from build123d import *

# Parameters (mm, degrees)
EXTRUDE_1_DEPTH      = 40
EXTRUDE_1_DEPTH_BACK = 5
SKETCH_2_W           = 36
SKETCH_2_H           = 37
CUT_EXTRUDE_1_DEPTH  = 50
SKETCH_5_W           = 36
SKETCH_5_H           = 5
CUT_EXTRUDE_4_DEPTH  = 43
SKETCH_9_R           = 1.025
CUT_EXTRUDE_5_DEPTH  = 45.5
SKETCH_10_W          = 3
SKETCH_10_H          = 8
EXTRUDE_4_DEPTH      = 10
SKETCH_11_W          = 3
SKETCH_11_H          = 18.5
EXTRUDE_5_DEPTH      = 10
SKETCH_12_R          = 1.05
CUT_EXTRUDE_6_DEPTH  = 10
SKETCH_13_R          = 1.05
CUT_EXTRUDE_7_DEPTH  = 63.5
FILLET_4_R           = 2
FILLET_5_R           = 2
FILLET_6_R           = 2
FILLET_7_R           = 2


with BuildPart() as part:
    # 草圖1 → 填料-伸長1 (new, two sides: drawn at the far end of the back side and taken through both)
    with BuildSketch(Plane.XY.offset(-EXTRUDE_1_DEPTH_BACK)):
        Polygon((-14.545454545, -28.090909091), (-15.545454545, -28.090909091), (-15.545454545, 16.909090909), (-14.545454545, 16.909090909), (25.454545455, 16.909090909), (26.454545455, 16.909090909), (26.454545455, -28.090909091), (25.454545455, -28.090909091), align=None)
    extrude(amount=EXTRUDE_1_DEPTH + EXTRUDE_1_DEPTH_BACK)

    # 草圖2 → 除料-伸長1 (cut)
    with BuildSketch(Plane(origin=(0, 16.909090909, 0), x_dir=(1, 0, 0), z_dir=(0, 1, 0))):
        with Locations((5.454545455, -21.5)):
            Rectangle(SKETCH_2_W, SKETCH_2_H)
    extrude(amount=-CUT_EXTRUDE_1_DEPTH, mode=Mode.SUBTRACT)

    # 草圖5 → 除料-伸長4 (cut)
    with BuildSketch(Plane(origin=(0, 16.909090909, 0), x_dir=(1, 0, 0), z_dir=(0, 1, 0))):
        with Locations((5.454545455, -0.5)):
            Rectangle(SKETCH_5_W, SKETCH_5_H)
    extrude(amount=-CUT_EXTRUDE_4_DEPTH, mode=Mode.SUBTRACT)

    # 草圖9 → 除料-伸長5 (cut)
    with BuildSketch(Plane.ZY.offset(15.545454545)):
        with Locations(Location((37, -25.090909091, 0), (0, 0, 180))):
            Circle(SKETCH_9_R)
        with Locations(Location((37, 13.909090909, 0), (0, 0, 180))):
            Circle(SKETCH_9_R)
    extrude(amount=-CUT_EXTRUDE_5_DEPTH, mode=Mode.SUBTRACT)

    # 草圖10 → 填料-伸長4 (add)
    with BuildSketch(Plane(origin=(0, 16.909090909, 0), x_dir=(1, 0, 0), z_dir=(0, 1, 0))):
        with Locations((-14.045454545, -17.5)):
            Rectangle(SKETCH_10_W, SKETCH_10_H)
        with Locations((24.954545455, -17.5)):
            Rectangle(SKETCH_10_W, SKETCH_10_H)
    extrude(amount=EXTRUDE_4_DEPTH)

    # 草圖11 → 填料-伸長5 (add)
    with BuildSketch(Plane(origin=(0, -28.090909091, 0), x_dir=(-1, 0, 0), z_dir=(0, -1, 0))):
        with Locations((-24.954545455, -30.75)):
            Rectangle(SKETCH_11_W, SKETCH_11_H)
        with Locations((-24.954545455, -4.25)):
            Rectangle(SKETCH_11_W, SKETCH_11_H)
        with Locations((14.045454545, -30.75)):
            Rectangle(SKETCH_11_W, SKETCH_11_H)
        with Locations((14.045454545, -4.25)):
            Rectangle(SKETCH_11_W, SKETCH_11_H)
    extrude(amount=EXTRUDE_5_DEPTH)

    # 草圖12 → 除料-伸長6 (cut)
    with BuildSketch(Plane(origin=(0, 0, 13.5), x_dir=(-1, 0, 0), z_dir=(0, 0, -1))):
        with Locations((-24.954545455, 21.909090909)):
            Circle(SKETCH_12_R)
        with Locations((14.045454545, 21.909090909)):
            Circle(SKETCH_12_R)
    extrude(amount=-CUT_EXTRUDE_6_DEPTH, mode=Mode.SUBTRACT)

    # 草圖13 → 除料-伸長7 (cut)
    with BuildSketch(Plane(origin=(0, 0, -5), x_dir=(-1, 0, 0), z_dir=(0, 0, -1))):
        with Locations((-24.954545455, -33.090909091)):
            Circle(SKETCH_13_R)
        with Locations((14.045454545, -33.090909091)):
            Circle(SKETCH_13_R)
    extrude(amount=-CUT_EXTRUDE_7_DEPTH, mode=Mode.SUBTRACT)

    # 圓角4
    # the kernel refuses this fillet: 2 mm, written as the material it takes off along each edge
    with BuildSketch(Plane(origin=(26.454545455, 21.909090909, -5), x_dir=(-1, 0, 0), z_dir=(0, -1, 0))) as fillet_4_piece_1:
        with BuildLine():
            CenterArc((FILLET_4_R, -FILLET_4_R), FILLET_4_R, 90, 90)
            Line((0, -FILLET_4_R), (0, 0))
            Line((0, 0), (FILLET_4_R, 0))
        make_face()
    extrude(amount=65, mode=Mode.SUBTRACT)

    # 圓角5
    # the kernel refuses this fillet: 2 mm, written as the material it takes off along each edge
    with BuildSketch(Plane(origin=(-15.545454545, 21.909090909, -5), x_dir=(0, 0, 1), z_dir=(0, -1, 0))) as fillet_5_piece_1:
        with BuildLine():
            CenterArc((FILLET_5_R, -FILLET_5_R), FILLET_5_R, 90, 90)
            Line((0, -FILLET_5_R), (0, 0))
            Line((0, 0), (FILLET_5_R, 0))
        make_face()
    extrude(amount=65, mode=Mode.SUBTRACT)

    # 圓角6
    # the kernel refuses this fillet: 2 mm, written as the material it takes off along each edge
    with BuildSketch(Plane(origin=(26.454545455, 21.909090909, 40), x_dir=(0, 0, -1), z_dir=(0, -1, 0))) as fillet_6_piece_1:
        with BuildLine():
            CenterArc((FILLET_6_R, -FILLET_6_R), FILLET_6_R, 90, 90)
            Line((0, -FILLET_6_R), (0, 0))
            Line((0, 0), (FILLET_6_R, 0))
        make_face()
    extrude(amount=65, mode=Mode.SUBTRACT)

    # 圓角7
    # the kernel refuses this fillet: 2 mm, written as the material it takes off along each edge
    with BuildSketch(Plane(origin=(-15.545454545, -43.090909091, 40), x_dir=(0, 0, -1), z_dir=(0, 1, 0))) as fillet_7_piece_1:
        with BuildLine():
            CenterArc((FILLET_7_R, -FILLET_7_R), FILLET_7_R, 90, 90)
            Line((0, -FILLET_7_R), (0, 0))
            Line((0, 0), (FILLET_7_R, 0))
        make_face()
    extrude(amount=65, mode=Mode.SUBTRACT)


solid = part.part
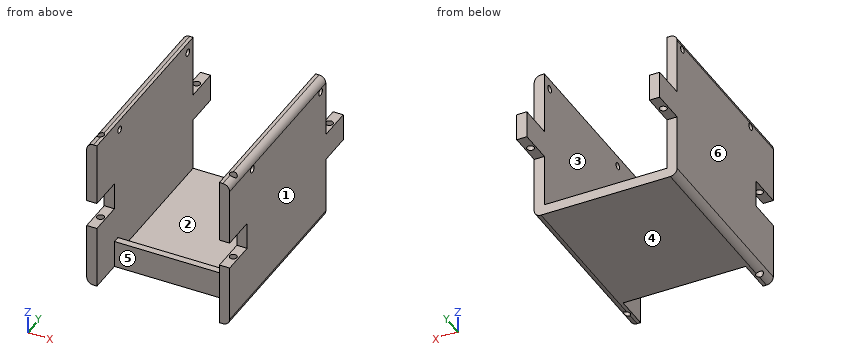
Build history of the part. All positions in model axes, mm. Face numbers are marked on the shaded views. A direction names the side the tool comes from. Round coordinates to 2 decimals unless told otherwise and drop trailing zeros. Loops run counter-clockwise (first coordinate to the right, second up) from the corner with the lowest first, then second, coordinate; pieces in that order, holes last. Notation, with made-up numbers: (24.5, 45) -> (53.5, 45) arc R22 cw to (53.5, 54) -> close; hole circle Ø10 at (30.5, 9). An arc over 180 degrees is marked (long way). Answer in a Markdown table with one row per item.
Item 1: Mould opens along X. For the marked faces 1, 2, 3 and 4 say: +X half, -X half, draft (parallel to the pull), parting line (faces both ways), or undercut.
Answers below:
| item | result |
|---|---|
| face 1 | +X half |
| face 2 | undercut |
| face 3 | undercut |
| face 4 | draft |
Item 2: Drill centre lines: L1, parallel to Y at x = -14, z = 37; L2, parallel to X at y = 7, z = 25.5; L3, parallel to Y at x = -13.85, z = 37. Where is each one in solid material? Low to high. Write a range as [from, to].
Answers below:
| item | result |
|---|---|
| L1 | y = [-38.09, -34.14], [-32.04, -26.12], [-24.07, 12.88], [14.93, 16.91] |
| L2 | x = [-15.55, -12.55], [23.45, 26.45] |
| L3 | y = [-38.09, -34.12], [-32.06, -26.12], [-24.07, 12.88], [14.93, 16.91] |
Item 3: Saw through at B-B (y = -19). Write the cut outline in (x, z), and give its area (3 significant figures).
Answers below:
| item | result |
|---|---|
| outline | (-15.55, -3) arc R2 ccw to (-13.55, -5) -> (24.45, -5) arc R2 ccw to (26.45, -3) -> (26.45, 38) arc R2 ccw to (24.45, 40) -> (23.45, 40) -> (23.45, -2) -> (-12.55, -2) -> (-12.55, 40) -> (-13.55, 40) arc R2 ccw to (-15.55, 38) -> close |
| area | 375 mm² |
Item 4: Saw through at C-C (x = -11). Write the cut outline in (y, z), and give its area (3 significant figures).
Answers below:
| item | result |
|---|---|
| outline | (-28.09, -5) -> (16.91, -5) -> (16.91, -2) -> (-26.09, -2) -> (-26.09, 3) -> (-28.09, 3) -> close |
| area | 145 mm² |
Item 5: Saw through at A-A (z = 32.5). Write the cut outline in (x, y), and give its area (3 significant figures).
Answers below:
| item | result |
|---|---|
| outline | (-15.55, -38.09) -> (-12.55, -38.09) -> (-12.55, 16.91) -> (-15.55, 16.91) -> close; (23.45, -38.09) -> (26.45, -38.09) -> (26.45, 16.91) -> (23.45, 16.91) -> close; hole circle Ø2.1 at (-14.05, -33.09); hole circle Ø2.1 at (24.95, -33.09) |
| area | 323 mm² |
Item 6: Pin check, flat tips, straight feed: pin 1 (2.5 mm diameter, centred on y = 13.91, z = 37, fed in from -X); pin 2 (3.5 mm diameter, centred on x = 25, y = 19.5, fed in from +Z); pin 3 (18 mm diameter, centred on x = -2.5, y = -0.5, fed in from +Z); pin 4 (5.5 mm diameter, centred on x = -4.5, z = 0.5, fed in from +Y). Stop position of each tip, or through.
Answers below:
| item | result |
|---|---|
| pin 1 | stops at x = -15.55 |
| pin 2 | stops at z = 21.5 |
| pin 3 | stops at z = -2 |
| pin 4 | stops at y = 16.91 |
Item 7: Which spindle directions (+Z, -Z, +X, -X, +Y, -Y) get a long thin tool onto all of the face, cutting with end or side? Do the marked faces 5 and 6. Say none if no direction does.
Answers below:
| item | result |
|---|---|
| face 5 | +Z, -Z, -Y |
| face 6 | +Z, -Z, -X, +Y, -Y |
